Autodesk Inventor part; units mm, degrees
ref_plane "YZ Plane" through (0, 0, 0) normal (1, 0, 0) x (0, 1, 0)
ref_plane "XZ Plane" through (0, 0, 0) normal (0, 1, 0) x (-1, 0, 0)
ref_plane "XY Plane" through (0, 0, 0) normal (0, 0, 1) x (1, 0, 0)
sketch "Skizze1" plane through (0, 0, 0) normal (0, 0, 1) x (1, 0, 0)
  line L0 (-21.5, 0) -> (21.5, 0) construction
  line L1 (-11.5, -4) -> (-17.5, -4)
  arc A0 (-17.5, 4) -> (-17.5, -4) centre (-17.5, 0) ccw
  line L2 (-17.5, 4) -> (-11.5, 4)
  line L3 (-6.2085, 2) -> (6.2085, 2)
  line L4 (11.5, 4) -> (17.5, 4)
  arc A1 (17.5, -4) -> (17.5, 4) centre (17.5, 0) ccw
  line L5 (17.5, -4) -> (11.5, -4)
  line L6 (-6.2085, -2) -> (6.2085, -2)
  arc A2 (11.5, -4) -> (6.2085, -2) centre (6.2085, -10) ccw
  arc A3 (-6.2085, -2) -> (-11.5, -4) centre (-6.2085, -10) ccw
  arc A4 (6.2085, 2) -> (11.5, 4) centre (6.2085, 10) ccw
  arc A5 (-11.5, 4) -> (-6.2085, 2) centre (-6.2085, 10) ccw
  point P0 (0, 0)
  point P1 (0, 0)
  dimension "d0" = 8
  dimension "d1" = 8
  dimension "d2" = 4
  dimension "d3" = 6
  dimension "d4" = 6
  dimension "d5" = 35
  dimension "d7" = 8
extrude "Extrusion1" add sketch "Skizze1" along normal blind 4
sketch "Skizze2" plane through (0, 0, 4) normal (0, 0, 1) x (1, 0, 0)
  arc A0 (-17.5, 4) -> (-17.5, -4) centre (-17.5, 0) ccw
  point P0 (0, 0)
hole "Bohrung1" at (-17.5, 0, 4) direction (0, 0, -1) diameter 4 end through all
sketch "Skizze3" plane through (0, 0, 4) normal (0, 0, 1) x (1, 0, 0)
  arc A0 (17.5, -4) -> (17.5, 4) centre (17.5, 0) ccw
  point P0 (0, 0)
hole "Bohrung2" at (17.5, 0, 4) direction (0, 0, -1) diameter 3 end through all
properties part number "Pleuel" material "Stahl, galvanisiert"
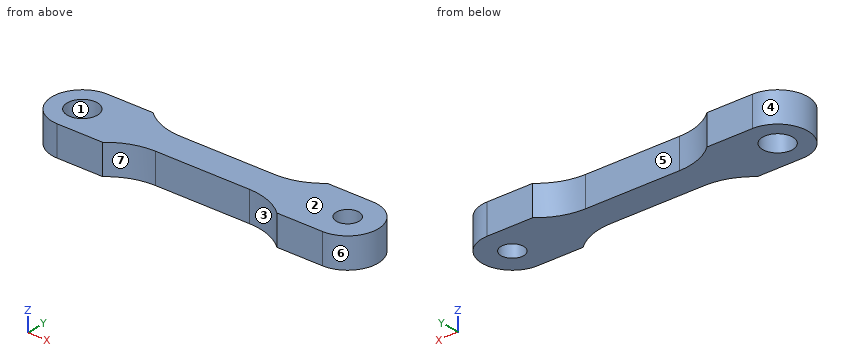
Geometry: final body of the model. Coordinates: model frame, mm. Face numbers are marked on the shaded views. A direction names the side the tool comes from. Round coordinates to 2 decimals unless told otherwise and drop trailing zeros. Loops run counter-clockwise (first coordinate to the right, second up) from the corner with the lowest first, then second, coordinate; pieces in that order, holes last.
Q1. Pin query (flat end, axial travel): P1, Ø2, axis at x = -2.5, z = 1.5, coming from the -Y side. Return the tip coordinate at first contact, or that it passes through.
Q2. Material intervals for L1, parallel to X at y = 0, z = 2.45; L2, parallel to Y at x = 17.5, z = 1.8; L3, parallel to Y at x = -17.5, z = 1.3, sorted ascending.
Q3. Section D-D on x = 17. Return loops of the section in (y, z).
Q4. Section C-C on x = -19. Return loops of the section in (y, z).
Q5. Section B-B on z = 0.9. Return loops of the section in (x, y), plus the area to 3 significant figures.
Q6. Access query for the marked faces 5, 6 and 7. Directions: +Z, -Z, +X, -X, +Y, -Y. A direction counts if a zero-diameter tool reaches every point of the face in a straight line with its end or side. Return the directions, or none.
Q7. Pull-direction query (Y, two-part tool) for the marked faces 1, 2, 3 and 4; classes: released by +Y, released by -Y, zero draft, split by the parting line, or undercut.
Q8. Section A-A on y = 0. Return loops of the section in (x, z), plus the area to 3 significant figures.
Evaluation:
1. P1: stops at y = -2
2. L1: x = -21.5 to -19.5, -15.5 to 16, 19 to 21.5
2. L2: y = -4 to -1.5, 1.5 to 4
2. L3: y = -4 to -2, 2 to 4
3. outline: (-4, 0) - (-1.41, 0) - (-1.41, 4) - (-4, 4) - close; (1.41, 0) - (4, 0) - (4, 4) - (1.41, 4) - close
4. outline: (-3.71, 0) - (-1.32, 0) - (-1.32, 4) - (-3.71, 4) - close; (1.32, 0) - (3.71, 0) - (3.71, 4) - (1.32, 4) - close
5. outline: (-17.5, -4) - (-11.5, -4) arc R8 cw to (-6.21, -2) - (6.21, -2) arc R8 cw to (11.5, -4) - (17.5, -4) arc R4 ccw to (17.5, 4) - (11.5, 4) arc R8 cw to (6.21, 2) - (-6.21, 2) arc R8 cw to (-11.5, 4) - (-17.5, 4) arc R4 ccw to start; hole circle Ø4 at (-17.5, 0); hole circle Ø3 at (17.5, 0)
5. area: 232 mm2
6. face 5: +Z, -Z, +Y
6. face 6: +Z, -Z, +X
6. face 7: +Z, -Z, -Y
7. face 1: undercut
7. face 2: zero draft
7. face 3: released by -Y
7. face 4: split by the parting line
8. outline: (-21.5, 0) - (-19.5, 0) - (-19.5, 4) - (-21.5, 4) - close; (-15.5, 0) - (16, 0) - (16, 4) - (-15.5, 4) - close; (19, 0) - (21.5, 0) - (21.5, 4) - (19, 4) - close
8. area: 144 mm2
